Here's how the part is built. I have some questions about the finished solid (model axes, mm). A direction names the side the tool comes from. Coordinates: 2 decimals unless noted, no trailing zeros. Order: outer loops, then holes, each group sorted by start corner. A loop starts at its lowest first (then second) coordinate and runs counter-clockwise, first axis right, second up.
Autodesk Inventor part; units mm, degrees
ref_plane "YZ Plane" through (0, 0, 0) normal (1, 0, 0) x (0, 1, 0)
ref_plane "XZ Plane" through (0, 0, 0) normal (0, 1, 0) x (-1, 0, 0)
ref_plane "XY Plane" through (0, 0, 0) normal (0, 0, 1) x (1, 0, 0)
sketch "Sketch1" plane through (0, 0, 0) normal (0, 0, 1) x (1, 0, 0)
  line L0 (37.223, 2.7469) -> (22.3469, -52.1291)
  arc A0 (12.6742, -52.5484) -> (22.3469, -52.1291) centre (17.4439, -50.8) ccw
  line L1 (12.6742, -52.5484) -> (-3.6199, -8.0984)
  arc A1 (-3.9302, -6.35) -> (-3.6199, -8.0984) centre (1.1498, -6.35) ccw
  line L2 (-3.9302, -6.35) -> (-3.9302, 6.35)
  arc A2 (-0.0144, 11.2948) -> (-3.9302, 6.35) centre (1.1498, 6.35) ccw
  arc A3 (20.8415, 2.2589) -> (20.2651, 2.9475) centre (20.209, 2.315) ccw
  line L3 (20.2651, 2.9475) -> (15.185, 3.3976)
  arc A4 (15.185, 3.3976) -> (14.4964, 2.8212) centre (15.1289, 2.7651) ccw
  line L4 (14.4964, 2.8212) -> (14.0462, -2.2589)
  arc A5 (14.0462, -2.2589) -> (14.6227, -2.9475) centre (14.6788, -2.315) ccw
  line L5 (14.6227, -2.9475) -> (19.7028, -3.3976)
  arc A6 (19.7028, -3.3976) -> (20.3914, -2.8212) centre (19.7589, -2.7651) ccw
  line L6 (20.3914, -2.8212) -> (20.8415, 2.2589)
  circle A7 centre (17.4439, -38.1) radius 5.08
  circle A8 centre (17.4439, -25.4) radius 2.1082
  circle A9 centre (17.4439, -12.7) radius 2.1082
  circle A10 centre (30.1439, 0) radius 2.1082
  circle A11 centre (17.4439, 12.7) radius 2.1082
  circle A12 centre (1.1498, 6.35) radius 2.1844
  circle A13 centre (1.1498, -6.35) radius 2.1844
  circle A14 centre (17.4439, -50.8) radius 2.0955
  line L7 (-0.0144, 11.2948) -> (3.3342, 11.2948) construction
  line L8 (3.3342, 11.2948) -> (7.5872, 13.6698) construction
  line L9 (7.5872, 13.6698) -> (12.3639, 16.3695) construction
  line L10 (12.3639, 16.3695) -> (17.4439, 17.5149) construction
  line L11 (17.4439, 17.5149) -> (26.2926, 14.8082) construction
  line L12 (26.2926, 14.8082) -> (32.2521, 11.2948) construction
  line L13 (32.2521, 11.2948) -> (37.9163, 7.1275) construction
  line L14 (37.9163, 7.1275) -> (37.223, 2.7469) construction
  spline S0 degree 4 poles (-0.0144, 11.2948) (3.3342, 11.2948) (7.5872, 13.6698) (12.3639, 16.3695) (17.4439, 17.5149) (26.2926, 14.8082) (32.2521, 11.2948) (37.9163, 7.1275) (37.223, 2.7469) knots 1 1 1 1 1 2 3 4 5 6 6 6 6 6
  point P0 (-3.9302, 6.35)
  point P1 (-3.9302, -6.35)
  point P2 (-3.6199, -8.0984)
  point P3 (12.6742, -52.5484)
  point P4 (21.7462, -53.5011)
  point P5 (20.8415, 2.2589)
  point P6 (20.3914, -2.8212)
  point P7 (14.6227, -2.9475)
  point P8 (14.4964, 2.8212)
  point P9 (20.2651, 2.9475)
  dimension "d0" = 4.3688
  dimension "d1" = 4.3688
  dimension "d2" = 4.2164
  dimension "d3" = 4.2164
  dimension "d5" = 4.2164
  dimension "d6" = 4.2164
  dimension "d7" = 10.16
  dimension "d8" = 4.191
extrude "Extrusion1" add sketch "Sketch1" along normal blind 1.524
properties part number "coffin-v2"
Q1. For faces 1 (the flat face through (4.64, -30.63, 0.75)), 2 (the flat face through (17.13, -3.17, 0.75)), which set-ups out of +Z, -Z, +X, -X, +Y, -Y let a thin tool reach every point of the face, with its end or its side?
Q2. If we section it at C-C on z = 1: Give the number of separate pieces and of enclosed holes in the cut face, then the cut area to 3 significant figures.
Q3. If we section it at A-A on y = -12.7: Write out the boundary of the cut face in (x, z).
Q4. If we section it at D-D on y = -25.4: Write out the boundary of the cut face in (x, z).
Q5. I need wall thicknesses on L1, parallel to Y at x = 20, z = 0.75; L2, parallel to X at y = -41.5, z = 1.05; L3, parallel to X at y = 13.5, z = 0.7. Which ranges of each line are inside material? Lowest first, please.
Q6. We'd pull the mould along Y, two halves only. Please class faces 3 (the cylindrical face through (17.17, -14.79, 0.75)), 4 (the cylindrical face through (-2.86, 9.47, 0.75)), 5 (the flat face through (16.7, -10.5, 1.524)): pulls with the +Y half, pulls with the -Y half, needs draft (parallel to the pull), parting line crosses it, or undercut.
Q7. If we section it at B-B on y = 0: Write out the boundary of the cut face in (x, z).
Reply:
1. face 1: +Z, -Z, -X, -Y
1. face 2: +Z, -Z
2. separate pieces: 1
2. enclosed holes: 9
2. area: 1,720 mm2
3. outline: (-1.93, 0) - (15.34, 0) - (15.34, 1.52) - (-1.93, 1.52) - close; (19.55, 0) - (33.04, 0) - (33.04, 1.52) - (19.55, 1.52) - close
4. outline: (2.72, 0) - (15.34, 0) - (15.34, 1.52) - (2.72, 1.52) - close; (19.55, 0) - (29.59, 0) - (29.59, 1.52) - (19.55, 1.52) - close
5. L1: y = -55.19 to -42.49, -33.71 to -3.35, 2.97 to 16.43
5. L2: x = 8.62 to 13.67, 21.22 to 25.23
5. L3: x = 7.3 to 15.49, 19.39 to 27.99
6. face 3: undercut
6. face 4: pulls with the +Y half
6. face 5: needs draft
7. outline: (-3.93, 0) - (14.25, 0) - (14.25, 1.52) - (-3.93, 1.52) - close; (20.64, 0) - (28.04, 0) - (28.04, 1.52) - (20.64, 1.52) - close; (32.25, 0) - (36.48, 0) - (36.48, 1.52) - (32.25, 1.52) - close
